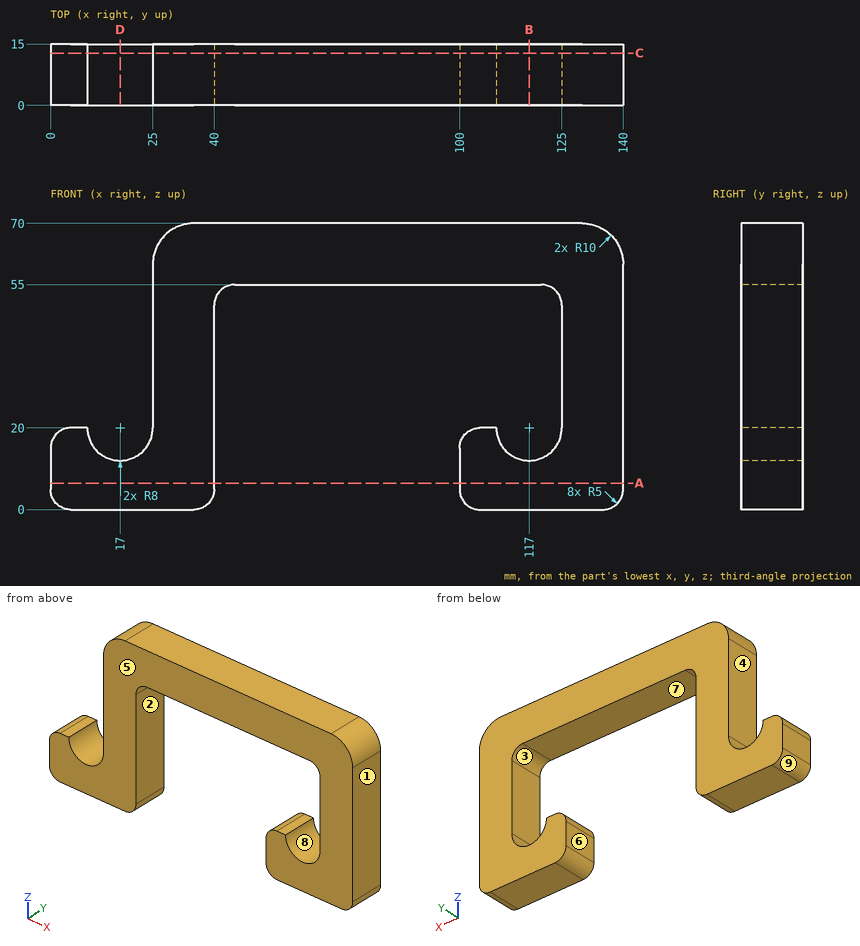
Geometry: see drawing. Coordinates: mm, zero at the bounding-box minimum. A direction names the side the tool comes from. Round coordinates to 2 decimals unless told otherwise and drop trailing zeros. Write each loop counter-clockwise with the first axis right and the second up, starting at its lowest first coordinate (ties: lowest second). Pieces come first, ordered by that corner, then holes.
1) Cut plane B-B (x = 117). Return the cut outline in (y, z), then the cut area to 3 significant figures.
2) Draft query along Z for the marked faces 6, 7, 8 and 9. Return one class per face: pulls with the +Z half, pulls with the -Z half, needs draft (parallel to the pull), parting line crosses it, or undercut.
3) Cut plane D-D (x = 17). Return the cut outline in (y, z), then the cut area to 3 significant figures.
4) Contact query for flat-ended pins moving along their axis: P1, Ø2, axis at x = 118.5, z = 13.5, coming from the +Y side; P2, Ø1.2, axis at x = 7, y = 11, coming from the +Z side; P3, Ø8, axis at x = 41, y = 2, coming from the -Z side; P4, Ø1.5, axis at y = 10, z = 35.5, coming from the -X side. Output: stop coordinate, or through.
5) Cut plane A-A (z = 6.5). Return the cut outline in (x, y), then the cut area to 3 significant figures.
6) Reachability of the marked faces 1, 2, 3, 4 and 5 from +Z, -Z, +X, -X, +Y, -Y: full face, straight path, thin tool, end or side. Return the list, or none.
7) Cut plane C-C (y = 12.75). Return the cut outline in (x, z).
8) Ray query, L1, parallel to X at y = 8.25, z = 9; L2, parallel to X at y = 12, z = 43; L3, parallel to X at y = 13.75, z = 16.5. Return the intervals inside material, ascending.
Geometry says:
1. outline: (0, 0) - (15, 0) - (15, 12) - (0, 12) - close; (0, 55) - (15, 55) - (15, 70) - (0, 70) - close
1. area: 405 mm2
2. face 6: needs draft
2. face 7: undercut
2. face 8: undercut
2. face 9: pulls with the -Z half
3. outline: (0, 0) - (15, 0) - (15, 12) - (0, 12) - close
3. area: 180 mm2
4. P1: passes through
4. P2: stops at z = 20
4. P3: stops at z = 0.42
4. P4: stops at x = 25
5. outline: (0, 0) - (40, 0) - (40, 15) - (0, 15) - close; (100, 0) - (140, 0) - (140, 15) - (100, 15) - close
5. area: 1,200 mm2
6. face 1: +Z, -Z, +X, +Y, -Y
6. face 2: -Z, +Y, -Y
6. face 3: +Y, -Y
6. face 4: +Z, -X, +Y, -Y
6. face 5: +Z, -Z, +X, -X, -Y
7. outline: (0, 5) arc R5 ccw to (5, 0) - (35, 0) arc R5 ccw to (40, 5) - (40, 50) arc R5 cw to (45, 55) - (120, 55) arc R5 cw to (125, 50) - (125, 20) arc R8 cw to (109, 20) - (105, 20) arc R5 ccw to (100, 15) - (100, 5) arc R5 ccw to (105, 0) - (135, 0) arc R5 ccw to (140, 5) - (140, 60) arc R10 ccw to (130, 70) - (35, 70) arc R10 ccw to (25, 60) - (25, 20) arc R8 cw to (9, 20) - (5, 20) arc R5 ccw to (0, 15) - close
8. L1: x = 0 to 40, 100 to 140
8. L2: x = 25 to 40, 125 to 140
8. L3: x = 0.23 to 9.81, 24.19 to 40, 100.23 to 109.81, 124.19 to 140
